Check sheet for the modelled part. Datum: model origin and axes. Units: mm. Face numbers are marked on the shaded views. Give positions to 0.01 mm unless a question says otherwise; leave off trailing zeros. Order: outer loops, then holes, each group sorted by start corner. A loop starts at its lowest first (then second) coordinate and runs counter-clockwise, first axis right, second up. Notation, with made-up numbers: (21, -37) -> (70, -37) arc R30 cw to (70, -9) -> close; hole circle Ø11 at (-2.75, 66). An arc over 180 degrees is marked (long way). Answer in a Markdown table with one row per item. Add a question column.
(1) Cross-section at A-A (x = 0). Record the cut outline in (y, z).
(2) Thickness scan on L1, parallel to Z at x = 0, y = 4; L2, parallel to X at y = 3.6, z = 7; L3, parallel to X at y = 3.35, z = -31. Record the ranges inside material, lowest first. Write a range as [from, to].
(3) Release check for a two-part mould opening along Z. For the marked faces 1, 2 and 3 record: released by +Z, released by -Z, zero draft, split by the parting line, or undercut.
(4) Cross-section at C-C (z = 31). Record the cut outline in (x, y), then the cut area to 3 significant figures.
(5) Cross-section at B-B (y = 1.1). Record the cut outline in (x, z), then the cut area to 3 significant figures.
(6) Cross-section at D-D (z = 17.5). Record the cut outline in (x, y).
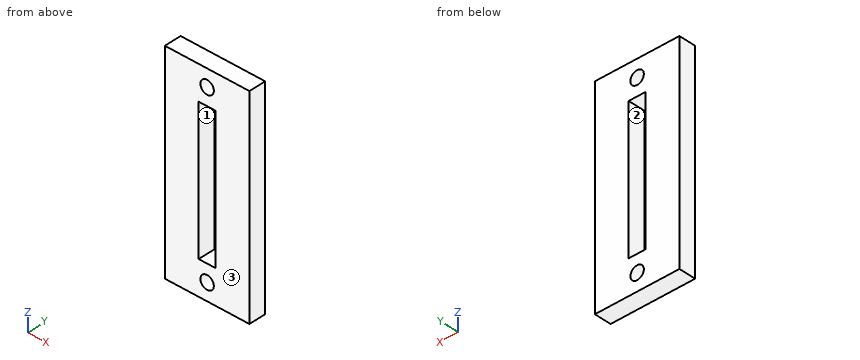
Autodesk Inventor part; units mm, degrees
ref_plane "YZ Plane" through (0, 0, 0) normal (1, 0, 0) x (0, 1, 0)
ref_plane "XZ Plane" through (0, 0, 0) normal (0, 1, 0) x (-1, 0, 0)
ref_plane "XY Plane" through (0, 0, 0) normal (0, 0, 1) x (1, 0, 0)
sketch "Boceto1" plane through (0, 0, 0) normal (0, 1, 0) x (-1, 0, 0)
  line L0 (-15, -37) -> (15, -37)
  line L1 (15, -37) -> (15, 37)
  line L2 (15, 37) -> (-15, 37)
  line L3 (-15, 37) -> (-15, -37)
  line L4 (-15, -37) -> (15, 37) construction
  line L5 (15, -37) -> (-15, 37) construction
  line L6 (-3, -25) -> (3, -25)
  line L7 (3, -25) -> (3, 25)
  line L8 (3, 25) -> (-3, 25)
  line L9 (-3, 25) -> (-3, -25)
  line L10 (-3, -25) -> (3, 25) construction
  line L11 (3, -25) -> (-3, 25) construction
  point P0 (0, 0)
  dimension "d2" = 6
  dimension "d3" = 50
  dimension "d4" = 12
  dimension "d5" = 12
extrude "Extrusión1" add sketch "Boceto1" along normal blind 6
sketch "Boceto2" plane through (0, 6, 0) normal (0, 1, 0) x (1, 0, 0)
  circle A0 centre (0, -31) radius 2.3812
  line L0 (-15, -37) -> (15, -37)
  point P0 (0, 0)
  dimension "d8" = 4.7625
  dimension "d9" = 6
extrude "Extrusión2" cut sketch "Boceto2" against normal through all
mirror "Simetría1" about plane through (0, 0, 0) normal (0, 0, 1) of "Extrusión2"
properties part number "sotenedor"
Answer below:
| question | item | result |
|---|---|---|
| 1 | outline | (0, -37) -> (6, -37) -> (6, -33.38) -> (0, -33.38) -> close; (0, -28.62) -> (6, -28.62) -> (6, -25) -> (0, -25) -> close; (0, 25) -> (6, 25) -> (6, 28.62) -> (0, 28.62) -> close; (0, 33.38) -> (6, 33.38) -> (6, 37) -> (0, 37) -> close |
| 2 | L1 | z = [-37, -33.38], [-28.62, -25], [25, 28.62], [33.38, 37] |
| 2 | L2 | x = [-15, -3], [3, 15] |
| 2 | L3 | x = [-15, -2.38], [2.38, 15] |
| 3 | face 1 | undercut |
| 3 | face 2 | undercut |
| 3 | face 3 | zero draft |
| 4 | outline | (-15, 0) -> (-2.38, 0) -> (-2.38, 6) -> (-15, 6) -> close; (2.38, 0) -> (15, 0) -> (15, 6) -> (2.38, 6) -> close |
| 4 | area | 151 mm² |
| 5 | outline | (-15, -37) -> (15, -37) -> (15, 37) -> (-15, 37) -> close; hole (-3, -25) -> (3, -25) -> (3, 25) -> (-3, 25) -> close; hole circle Ø4.76 at (0, -31); hole circle Ø4.76 at (0, 31) |
| 5 | area | 1,880 mm² |
| 6 | outline | (-15, 0) -> (-3, 0) -> (-3, 6) -> (-15, 6) -> close; (3, 0) -> (15, 0) -> (15, 6) -> (3, 6) -> close |
